The figure shows three views and two pictorial views of one solid part (mm, origin at its lowest corner). Answer the questions. Coordinates: 2 decimals unless noted, no trailing zeros. Order: outer loops, then holes, each group sorted by start corner. A loop starts at its lowest first (then second) coordinate and runs counter-clockwise, first axis right, second up.
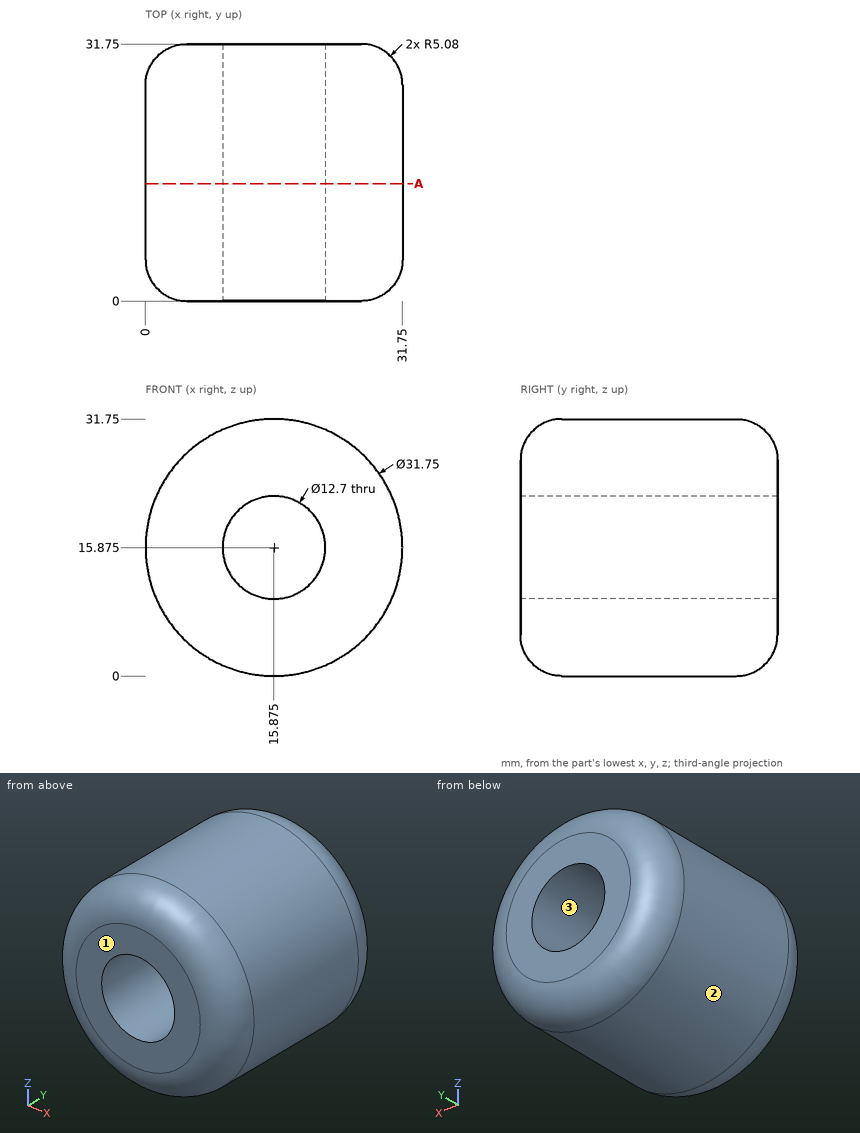
Q1. Determine the mould class of the marked faces 1, 2 and 3 for opening direction X: +X half, -X half, draft (parallel to the pull), parting line (faces both ways), or undercut.
Q2. The part is cut by section A-A, the plane y = 14.5. Determine the outline of the cut face in (x, z) (3 decimals), then the cut area to 3 significant figures.
Q3. Straight lines are drawn through the part: L1, parallel to X at y = 24.5, z = 13.5; L2, parallel to X at y = 14, z = 12.5; L3, parallel to Z at x = 18.5, y = 11.5. For each, find the intervals that lie inside material, in ascending order.
Q4. Each of these flat-tipped pins is pushed along its axis until it touches: P1, Ø4, axis at x = 26, y = 20, coming from the +Z side; P2, Ø1, axis at x = 24, y = 26.5, coming from the +Z side; P3, Ø4, axis at y = 11, z = 23.5, coming from the -X side. Where does it stop, or does it pass through?
Computed values:
1. face 1: draft
1. face 2: parting line
1. face 3: undercut
2. outline: circle Ø31.75 at (15.875, 15.875); hole circle Ø12.7 at (15.875, 15.875)
2. area: 665 mm2
3. L1: x = 0.18 to 9.99, 21.76 to 31.57
3. L2: x = 0.36 to 10.5, 21.25 to 31.39
3. L3: z = 0.22 to 10.09, 21.66 to 31.53
4. P1: stops at z = 29.51
4. P2: stops at z = 29.8
4. P3: stops at x = 1.03
